from build123d import *

# Parameters (mm, degrees)
F0_R     = 49.507556
F1_DEPTH = 50.8
F2_SIZE  = 5.08
F3_SIZE  = 5.08


with BuildPart() as f1:
    # F0 (on Top) → F1 (new body)
    with BuildSketch(Plane.XY):
        Circle(F0_R)
    extrude(amount=F1_DEPTH)

    # F2
    f2_edges = [f1.edges().sort_by_distance(p)[0] for p in [
        (-49.507556, 0, 50.8),
        (-49.507556, 0, 0),
    ]]
    chamfer(f2_edges, length=F2_SIZE)

    # F3
    f3_edges = [f1.edges().sort_by_distance(p)[0] for p in [
        (-44.427556, 0, 50.8),
    ]]
    chamfer(f3_edges, length=F3_SIZE)


solid = f1.part
Read the model definition and answer for the solid it produces. Units are mm, in the model's axes. Coordinates: 2 decimals unless noted, no trailing zeros. Loops run counter-clockwise (first coordinate to the right, second up) from the corner with the lowest first, then second, coordinate; pieces in that order, holes last. Notation, with made-up numbers: (20, 67) -> (63, 67) arc R29 ccw to (63, 88) -> close; hole circle Ø10 at (67, 37.25). An arc over 180 degrees is marked (long way). Answer in a Markdown table with one row per item.
Item 1: Each of these flat-tipped pins is pushed along its axis until it touches: P1, Ø5, axis at x = 38, z = 37.5, coming from the -Y side; P2, Ø1, axis at y = -38, z = 10, coming from the +X side; P3, Ø6, axis at x = 32, z = 17, coming from the +Y side. Where does it stop, or does it pass through?
Returned:
| item | result |
|---|---|
| P1 | stops at y = -34.51 |
| P2 | stops at x = 32.32 |
| P3 | stops at y = 40.12 |
Item 2: A cutting plane is placed at A-A on z = 15.5. Determine the outline of the cut face in (x, y).
Returned:
| item | result |
|---|---|
| outline | circle Ø99.02 at (0, 0) |
Item 3: Straight lines are drawn through the part: line 1 along Z through (x, y) = (-18, 35); line 2 along X through (y, z) = (-1, 15); line 3 along Y through (x, z) = (40, 36). For each, find the intervals that lie inside material, in ascending order. Write a range as [from, to].
Returned:
| item | result |
|---|---|
| line 1 | z = [0, 50.8] |
| line 2 | x = [-49.5, 49.5] |
| line 3 | y = [-29.17, 29.17] |
